```python
from build123d import *

# Parameters (mm, degrees)
F0_W      = 45
F0_H      = 15
F1_DEPTH  = 7.5
F2_W      = 50
F2_H      = 25
F3_DEPTH  = 20
F5_DEPTH  = 25
F7_DEPTH  = 25
F8_W      = 25
F8_H      = 20
F9_DEPTH  = 2
F11_W     = 5
F11_H     = 5
F13_W     = 5
F13_H     = 5
F15_R     = 10
F16_DEPTH = 3
F17_R     = 10
F18_DEPTH = 3
F19_R     = 2.5
F20_DEPTH = 3
F21_R     = 2.5
F22_DEPTH = 3


# Not quite as in the source:
# - a pattern or mirror of a feature is missing from the dataset's text; its kind, count and spacing are read off the source's solid


with BuildPart() as f1:
    # F0 (on Top) → F1 (new body, symmetric)
    with BuildSketch(Plane.XY):
        Rectangle(F0_W, F0_H)
    extrude(amount=F1_DEPTH, both=True)

    # F2 (on face) → F3 (join)
    with BuildSketch(Plane.XY.offset(7.5)):
        Rectangle(F2_W, F2_H)
    extrude(amount=F3_DEPTH)

    # F4 (on face) → F5 (cut, through all)
    with BuildSketch(Plane.XZ.offset(12.5)):
        Polygon((25, 27.5), (12.5, 27.5), (15, 25.0505102572), (25, 25.0505102572), align=None)
    extrude(amount=-F5_DEPTH, mode=Mode.SUBTRACT)

    # F6 (on face) → F7 (cut, through all)
    with BuildSketch(Plane.XZ.offset(12.5)):
        Polygon((-25, 27.5), (-25, 21.2550020016), (-22, 21.2550020016), (-17, 27.5), align=None)
    extrude(amount=-F7_DEPTH, mode=Mode.SUBTRACT)

    # F8 (on face) → F9 (join)
    with BuildSketch(Plane.XY.offset(27.5)):
        with Locations((-2, 0)):
            Rectangle(F8_W, F8_H)
    extrude(amount=F9_DEPTH)

    # F11 (on Front) → F12 (revolve)
    with BuildSketch(Plane.XZ):
        with Locations((25, -2.5)):
            Rectangle(F11_W, F11_H)
    revolve(axis=Axis((-8.4795374423, 0, 0), (-1, 0, 0)))

    # F13 (on Front) → F14 (revolve)
    with BuildSketch(Plane.XZ):
        with Locations((-25, -2.5)):
            Rectangle(F13_W, F13_H)
    revolve(axis=Axis((-8.4795374423, 0, 0), (-1, 0, 0)))

    # F15 (on face) → F16 (join)
    with BuildSketch(Plane.XZ.offset(7.5)):
        with Locations((-12.5, -3.5)):
            Circle(F15_R)
    f16 = extrude(amount=F16_DEPTH)

    # F16_copies: F16 across plane
    add(f16.mirror(Plane.ZX))

    # F17 (on face) → F18 (join)
    with BuildSketch(Plane.XZ.offset(7.5)):
        with Locations((12.5, -3.5)):
            Circle(F17_R)
    f18 = extrude(amount=F18_DEPTH)

    # F18_copies: F18 across plane
    add(f18.mirror(Plane.ZX))

    # F19 (on face) → F20 (join)
    with BuildSketch(Plane.XZ.offset(10.5)):
        with Locations((-12.5, -3.5)):
            Circle(F19_R)
    f20 = extrude(amount=F20_DEPTH)

    # F20_copies: F20 across plane
    add(f20.mirror(Plane.ZX))

    # F21 (on face) → F22 (join)
    with BuildSketch(Plane.XZ.offset(10.5)):
        with Locations((12.5, -3.5)):
            Circle(F21_R)
    f22 = extrude(amount=F22_DEPTH)

    # F22_copies: F22 across plane
    add(f22.mirror(Plane.ZX))

    # F23 (on Front) → F24 (revolve)
    with BuildSketch(Plane.XZ):
        with BuildLine():
            Line((-27.5, 0), (-27.5, 5))
            ThreePointArc((-27.5, 5), (-31.0355339059, 3.5355339059), (-32.5, 0))
            Line((-32.5, 0), (-27.5, 0))
        make_face()
    f24 = revolve(axis=Axis((-30, 0, 0), (1, 0, 0)))

    # F24_copies: F24 across plane
    add(f24.mirror(Plane(origin=(0, 0, 0), x_dir=(0, 0, 1), z_dir=(1, 0, 0))))


solid = f1.part
```
For this review, take the finished solid that the model builds, in its own axes (mm). A direction names the side the tool comes from. Round coordinates to 2 decimals unless told otherwise and drop trailing zeros. Write each loop counter-clockwise with the first axis right and the second up, starting at its lowest first coordinate (ties: lowest second). Pieces come first, ordered by that corner, then holes. Notation, with made-up numbers: (9.25, 8.5) -> (41.25, 8.5) arc R22 ccw to (41.25, 33.5) -> close; hole circle Ø7 at (5, 63). An arc over 180 degrees is marked (long way). One line per question, with ' | ' between items. Start each with the question number.
1) Mouldability with a two-part tool opening along X and no side actions: class faces 1 (the flat face through (13.732, -0.175, 26.292)), 2 (the flat face through (0, -7.5, 3)), 3 (the flat face through (20, 0, 25.051)) as +X half, -X half, draft (parallel to the pull), parting line (faces both ways), or undercut.
2) Add section B-B (x = 1). Write out the cut boundary in (y, z).
3) For pin 1 Ø8 at (y, z) = (2, 22) entering from -X; pin 2 Ø10 at (x, z) = (-2, 10.5) entering from -Y; pin 3 Ø9 at (y, z) = (-5, 14.5) entering from +X, all flat-tipped, find the tip position at first contact; note any pin that passes through.
4) Add section D-D (y = 0). Write out the cut boundary in (x, z) (3 decimals), and give its area (3 significant figures).
5) Machinability: for faces 4 (the flat face through (-2, -10, 28)), 5 (the flat face through (15, 10.5, -6)), 6 (the flat face through (-24, 0, 21.255)), 7 (the flat face through (-13, -7.5, -10)), which of the approach directions +Z, -Z, +X, -X, +Y, -Y give a long, thin tool a straight path to every point of the face, cutting with its end or side? Answer none if there is none.
6) Add section C-C (z = 8.5). Write out the cut boundary in (x, y).
7) Wall thickness on line 1 along X through (y, z) = (8, -7.5); line 2 along Z through (x, y) = (-23, 9.25) (3 decimals); line 3 along Y through (x, z) = (-4, 5.5): over which ranges is each line inside the solid? List them lowest first.
8) Add section A-A (y = 5.75). Write out the cut boundary in (x, z) (3 decimals), and give its area (3 significant figures).
Reported:
1) face 1: +X half | face 2: undercut | face 3: draft
2) outline: (-12.5, 7.5) -> (-7.5, 7.5) -> (-7.5, -7.5) -> (7.5, -7.5) -> (7.5, 7.5) -> (12.5, 7.5) -> (12.5, 27.5) -> (10, 27.5) -> (10, 29.5) -> (-10, 29.5) -> (-10, 27.5) -> (-12.5, 27.5) -> close
3) pin 1: stops at x = -25 | pin 2: stops at y = -12.5 | pin 3: stops at x = 25
4) outline: (-27.5, -5) -> (-22.5, -5) -> (-22.5, -7.5) -> (22.5, -7.5) -> (22.5, -5) -> (27.5, -5) arc R5 ccw to (27.5, 5) -> (22.5, 5) -> (22.5, 7.5) -> (25, 7.5) -> (25, 25.051) -> (15, 25.051) -> (12.5, 27.5) -> (10.5, 27.5) -> (10.5, 29.5) -> (-14.5, 29.5) -> (-14.5, 27.5) -> (-17, 27.5) -> (-22, 21.255) -> (-25, 21.255) -> (-25, 7.5) -> (-22.5, 7.5) -> (-22.5, 5) -> (-27.5, 5) arc R5 ccw to start | area: 1,840 mm²
5) face 4: +Z, +X, -X, -Y | face 5: +Y | face 6: +Z, -X, +Y, -Y | face 7: -Z, +X, -X
6) outline: (-25, -12.5) -> (25, -12.5) -> (25, 12.5) -> (-25, 12.5) -> close
7) line 1: x = -21.67 to -3.33, 3.33 to 21.67 | line 2: z = 7.5 to 21.255 | line 3: y = -7.5 to 7.5
8) outline: (-25, 7.5) -> (-22.5, 7.5) -> (-22.5, -7.5) -> (22.5, -7.5) -> (22.5, 7.5) -> (25, 7.5) -> (25, 25.051) -> (15, 25.051) -> (12.5, 27.5) -> (10.5, 27.5) -> (10.5, 29.5) -> (-14.5, 29.5) -> (-14.5, 27.5) -> (-17, 27.5) -> (-22, 21.255) -> (-25, 21.255) -> close | area: 1,660 mm²
